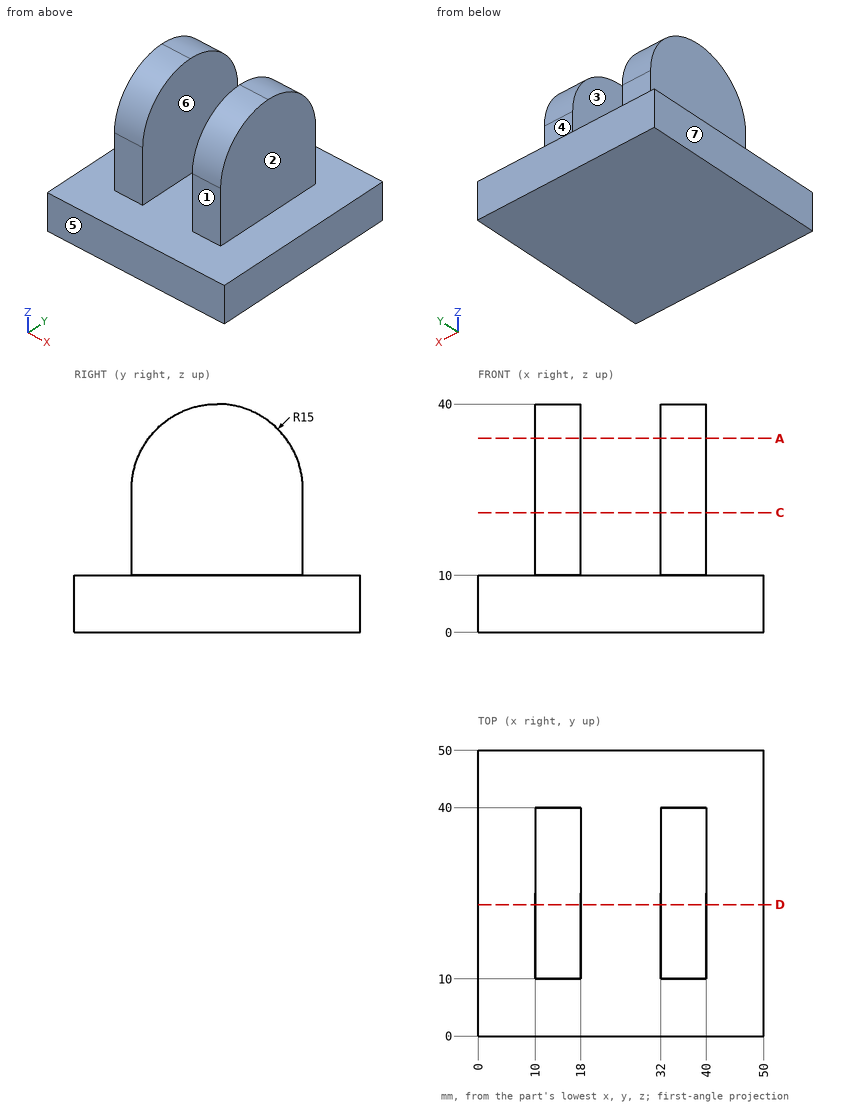
For this review, use the dimensioned drawing (mm, ordinates from the lowest corner) and the shaded views. A direction names the side the tool comes from. Give positions to 0.01 mm unless a question says otherwise; leave off trailing zeros. Order: outer loops, then holes, each group sorted by start corner. A loop starts at its lowest first (then second) coordinate and runs counter-clockwise, first axis right, second up.
1. Mouldability with a two-part tool opening along X and no side actions: class the marked faces 5, 6 and 7 as +X half, -X half, draft (parallel to the pull), parting line (faces both ways), or undercut.
Solution:
face 5: draft
face 6: undercut
face 7: -X half
2. Add section C-C, the plane z = 21. State the section outline as (x, y) points, then the cut area to 3 significant figures.
Solution:
outline: (10, 10) - (18, 10) - (18, 40) - (10, 40) - close; (32, 10) - (40, 10) - (40, 40) - (32, 40) - close
area: 480 mm2
3. Add section D-D, the plane y = 23. State the section outline as (x, z) points.
Solution:
outline: (0, 0) - (50, 0) - (50, 10) - (40, 10) - (40, 39.87) - (32, 39.87) - (32, 10) - (18, 10) - (18, 39.87) - (10, 39.87) - (10, 10) - (0, 10) - close
4. For pin 1 Ø4 at (x, z) = (34.5, 20) entering from -Y; pin 2 Ø6.5 at (x, z) = (14.5, 20) entering from +Y; pin 3 Ø3 at (x, z) = (39, 30) entering from -Y, all flat-tipped, find the tip position at first contact; note any pin that passes through.
Solution:
pin 1: stops at y = 10
pin 2: stops at y = 40
pin 3: stops at y = 10.41
5. Tool access review of the marked faces 1, 2, 3 and 4: name each direction out of +Z, -Z, +X, -X, +Y, -Y from which nothing blocks a thin tool from reaching the whole face with its end or side.
Solution:
face 1: +Z, +X, -X, -Y
face 2: +Z, +X, +Y, -Y
face 3: +Z, +Y, -Y
face 4: +Z, +X, -X, +Y
6. Add section A-A, the plane z = 34. State the section outline as (x, y) points.
Solution:
outline: (10, 13) - (18, 13) - (18, 37) - (10, 37) - close; (32, 13) - (40, 13) - (40, 37) - (32, 37) - close
7. To check wall thickness, follow L1, parallel to X at y = 18, z = 19.5; L2, parallel to Z at x = 35, y = 41; L3, parallel to Y at x = 33, z = 12. State the ranges of each line that lie inside material, in increasing order.
Solution:
L1: x = 10 to 18, 32 to 40
L2: z = 0 to 10
L3: y = 10 to 40
